from build123d import *

# Parameters (mm, degrees)
BOSS_EXTRUDE1_DEPTH = 3


with BuildPart() as part:
    # Model → Boss-Extrude1 (new body)
    with BuildSketch(Plane.XY):
        with BuildLine():
            Line((1255.301037795, 443.027781841), (1294.701037823, 443.027781841))
            Line((1294.701037823, 443.027781841), (1294.701037823, 553.849315832))
            add(Edge.make_bspline(
                [(1294.701037823, 553.849315832), (987.9659757, 523.139532485), (557.602899882, 467.780280961), (240.864040275, 415.199018527), (137.973344874, 389.690933183), (94.901037796, 377.220662508)],
                knots=[0.108777165, 0.108777165, 0.108777165, 0.108777165, 0.189662497, 0.216203451, 0.238160454, 0.238160454, 0.238160454, 0.238160454], degree=3))
            Line((94.901037796, 377.220662508), (94.901037796, 188.610331254))
            Line((94.901037796, 188.610331254), (97.901037796, 188.610331254))
            Line((97.901037796, 188.610331254), (97.901037796, 0))
            Line((97.901037796, 0), (253.901037796, 0))
            Line((253.901037796, 0), (253.901037796, 188.610331254))
            Line((253.901037796, 188.610331254), (256.901037795, 188.610331254))
            Line((256.901037795, 188.610331254), (256.901037795, 0))
            Line((256.901037795, 0), (412.901037795, 0))
            Line((412.901037795, 0), (412.901037795, 188.610331254))
            Line((412.901037795, 188.610331254), (415.901037795, 188.610331254))
            Line((415.901037795, 188.610331254), (415.901037795, 0))
            Line((415.901037795, 0), (571.901037795, 0))
            Line((571.901037795, 0), (571.901037795, 188.610331254))
            Line((571.901037795, 188.610331254), (574.901037795, 188.610331254))
            Line((574.901037795, 188.610331254), (574.901037795, 0))
            Line((574.901037795, 0), (730.901037795, 0))
            Line((730.901037795, 0), (730.901037795, 188.610331254))
            Line((730.901037795, 188.610331254), (733.901037795, 188.610331254))
            Line((733.901037795, 188.610331254), (733.901037795, 0))
            Line((733.901037795, 0), (889.901037795, 0))
            Line((889.901037795, 0), (889.901037795, 188.610331254))
            Line((889.901037795, 188.610331254), (892.901037795, 188.610331254))
            Line((892.901037795, 188.610331254), (892.901037795, 0))
            Line((892.901037795, 0), (1048.901037796, 0))
            Line((1048.901037796, 0), (1048.901037796, 188.610331254))
            Line((1048.901037796, 188.610331254), (1051.901037795, 188.610331254))
            Line((1051.901037795, 188.610331254), (1051.901037795, 0))
            Line((1051.901037795, 0), (1207.901037796, 0))
            Line((1207.901037796, 0), (1207.901037796, 188.610331254))
            Line((1207.901037796, 188.610331254), (1210.901037796, 188.610331254))
            Line((1210.901037796, 188.610331254), (1210.901037796, 0))
            Line((1210.901037796, 0), (1294.701037796, 0))
            Line((1294.701037796, 0), (1294.701037796, 232.227781841))
            Line((1294.701037796, 232.227781841), (1255.301037795, 232.227781841))
            Line((1255.301037795, 232.227781841), (1255.301037795, 212.230413534))
            ThreePointArc((1255.301037795, 212.230413534), (1224.501037792, 242.627781841), (1255.301037795, 273.025150148))
            Line((1255.301037795, 273.025150148), (1255.301037795, 253.027781841))
            Line((1255.301037795, 253.027781841), (1294.701037796, 253.027781841))
            Line((1294.701037796, 253.027781841), (1294.701037796, 422.227781841))
            Line((1294.701037796, 422.227781841), (1255.301037795, 422.227781841))
            Line((1255.301037795, 422.227781841), (1255.301037795, 402.230413534))
            ThreePointArc((1255.301037795, 402.230413534), (1224.501037792, 432.627781841), (1255.301037795, 463.025150148))
            Line((1255.301037795, 463.025150148), (1255.301037795, 443.027781841))
        make_face()
    extrude(amount=BOSS_EXTRUDE1_DEPTH)


solid = part.part
Geometry check sheet. Reference: the model listing, model coordinates, mm. Round coordinates to 2 decimals unless told otherwise and drop trailing zeros. Answer in a Markdown table with one row per item.
(1) Draft check along Y on faces 1 (the face through (686, 219, 3)), 2 (the face through (1224.51, 241.95, 1.48)), 3 (the face through (1224.51, 431.95, 1.48)). Enter one of: released by +Y, released by -Y, zero draft, split by the parting line, or undercut.
Responses:
| item | result |
|---|---|
| face 1 | zero draft |
| face 2 | undercut |
| face 3 | undercut |
(2) Go/stop test with flat-tipped pins: P1, Ø8, axis at x = 1014, y = 265.5, coming from the -Z side; P2, Ø0.9, axis at x = 255.5, z = 1, coming from the -Y side; P3, Ø1.5, axis at y = 130.5, z = 1, coming from the -X side. Record where each tip stops, or that it passes through.
Responses:
| item | result |
|---|---|
| P1 | stops at z = 0 |
| P2 | stops at y = 188.61 |
| P3 | stops at x = 97.9 |
(3) Scan lines: probe 1 along X at (y, z) = (246.5, 1.7); probe 2 along X at (y, z) = (261.5, 2.6); probe 3 along Y at (x, z) = (1004.5, 2.1). Record each from-to range of solid material in increasing order. Write a range as from..to.
Responses:
| item | result |
|---|---|
| probe 1 | x = 94.9..1224.75 |
| probe 2 | x = 94.9..1231.07, 1255.3..1294.7 |
| probe 3 | y = 0..522.27 |
